```python
from build123d import *

# Parameters (mm, degrees)
F0_R     = 1.25
F0_R_2   = 5.5
F1_DEPTH = 1.5
F2_R     = 5


with BuildPart() as f1:
    # F0 (on Top) → F1 (new body)
    with BuildSketch(Plane.XY):
        with BuildLine():
            ThreePointArc((0, -15), (8.2826006835, 0), (0, 15))
            ThreePointArc((0, 15), (-8.2826006835, 0), (0, -15))
        make_face()
        with Locations((0, -10)):
            Circle(F0_R, mode=Mode.SUBTRACT)
        Circle(F0_R_2, mode=Mode.SUBTRACT)
        with Locations((0, 10)):
            Circle(F0_R, mode=Mode.SUBTRACT)
    extrude(amount=F1_DEPTH)

    # F2
    f2_edges = [f1.edges().sort_by_distance(p)[0] for p in [
        (0, -15, 0.75),
        (0, 15, 0.75),
    ]]
    fillet(f2_edges, radius=F2_R)


solid = f1.part
```
The listing builds one solid part. Answer for the finished solid, in the listing's coordinates (mm). Coordinates: 2 decimals unless noted, no trailing zeros. Write each loop counter-clockwise with the first axis right and the second up, starting at its lowest first coordinate (ties: lowest second). Pieces come first, ordered by that corner, then holes. Notation, with made-up numbers: M 45.5,-13 L 90.5,-13 A19 ccw 90.5,13 Z; hole C 24,74.5 d3. An arc over 180 degrees is marked long. Use a Markdown table: item, result. Add a question column.
1. Section B-B (x = 0) is taken. Count the separate pieces of the cut face and the enclosed holes in it, plus the area to 3 significant figures.
2. Given P1, Ø3, axis at x = 0, y = 10, coming from the +Z side, flat-ended and moving along its own axis, determine where the tip first touches the part or whether it passes through.
3. Straight lines are drawn through the part: line 1 along Y through (x, z) = (0, 0.4); line 2 along X through (y, z) = (4.75, 1.15); line 3 along Y through (x, z) = (1.5, 0.1). For each, find the intervals that lie inside material, in ascending order. Write a range as [from, to].
4. For a pull along Y with two mould halves and no side action, classify faces 1 (the flat face through (0, -6, 1.5)), 2 (the cylindrical face through (-1.19, -5.37, 0.74)), 3 (the cylindrical face through (8.28, -0.18, 0.74)) as +Y half, -Y half, draft (parallel to the pull), parting line (faces both ways), or undercut.
5. Section D-D (y = -10) is taken. Give the vertices of the cut face in (x, z), plus the area to 3 significant figures.
6. Section A-A (y = 0) is taken. Give the vertices of the cut face in (x, z), plus the area to 3 significant figures.
Data:
| question | item | result |
|---|---|---|
| 1 | separate pieces | 4 |
| 1 | enclosed holes | 0 |
| 1 | area | 16.6 mm2 |
| 2 | P1 | stops at z = 1.5 |
| 3 | line 1 | y = [-13.53, -11.25], [-8.75, -5.5], [5.5, 8.75], [11.25, 13.53] |
| 3 | line 2 | x = [-7.63, -2.77], [2.77, 7.63] |
| 3 | line 3 | y = [-13.3, -5.29], [5.29, 13.3] |
| 4 | face 1 | draft |
| 4 | face 2 | undercut |
| 4 | face 3 | parting line |
| 5 | outline | M -5.19,0 L -1.25,0 L -1.25,1.5 L -5.19,1.5 Z; M 1.25,0 L 5.19,0 L 5.19,1.5 L 1.25,1.5 Z |
| 5 | area | 11.8 mm2 |
| 6 | outline | M -8.28,0 L -5.5,0 L -5.5,1.5 L -8.28,1.5 Z; M 5.5,0 L 8.28,0 L 8.28,1.5 L 5.5,1.5 Z |
| 6 | area | 8.35 mm2 |
